Check sheet for the modelled part. Datum: model origin and axes. Units: mm. A direction names the side the tool comes from. Round coordinates to 2 decimals unless told otherwise and drop trailing zeros. Loops run counter-clockwise (first coordinate to the right, second up) from the corner with the lowest first, then second, coordinate; pieces in that order, holes last. Notation, with made-up numbers: (86, -36.5) -> (120, -36.5) arc R25 ccw to (120, -11.5) -> close; hole circle Ø10 at (-0.75, 68.25). An arc over 180 degrees is marked (long way). One line per item, written item: value. Start each with the question number.
1. Go/stop test with flat-tipped pins: pin 1 (4 mm diameter, centred on x = -10.5, y = 9, fed in from -Z); pin 2 (10 mm diameter, centred on x = 7.5, z = -32, fed in from -Y); pin 3 (6 mm diameter, centred on x = -111.5, y = 8.5, fed in from +Z); pin 4 (6.5 mm diameter, centred on x = -91.5, y = 6, fed in from -Z). Record where each tip stops, or that it passes through.
2. Set-up check for faces 1 (the face through (-104, 6, -19.05)), 2 (the face through (104, 6, 19.05)), 3 (the face through (137.218, 6.261, -35.684)): record each of +Z, -Z, +X, -X, +Y, -Y from which the full face is reachable in a straight line by a thin tool's end or side.
3. Cross-section at D-D on x = -16. Record the cut outline in (y, z), then the cut area to 3 significant figures.
4. Cross-section at A-A on z = 23. Record the cut outline in (x, y).
5. Cross-section at B-B on y = 5.25. Record the cut outline in (x, z).
6. Material ranges on L1, parallel to Z at x = -41.5, y = 5.5; L2, parallel to X at y = 11.25, z = 41; L3, parallel to Z at x = 71, y = 8.5, recorded low to high.
7. Release check for a two-part mould opening along X. For faces 4 (the face through (-2, 0, -1)), 5 (the face through (55.31, 6.26, -27.41)), 6 (the face through (152.4, 6, -12)) record: +X half, -X half, draft (parallel to the pull), parting line (faces both ways), or undercut.
8. Cross-section at C-C on z = -23.5. Record the cut outline in (x, y), then the cut area to 3 significant figures.
from build123d import *

# Parameters (mm, degrees)
SKETCH1_R           = 38.1
BOSS_EXTRUDE1_DEPTH = 12.7


with BuildPart() as part:
    # Sketch1 → Boss-Extrude1 (new body)
    with BuildSketch(Plane(origin=(0, 0, 0), x_dir=(1, 0, 0), z_dir=(0, 1, 0))):
        with BuildLine():
            Line((-57.15762, 19.05), (-152.4, 19.05))
            Line((-152.4, 19.05), (-152.4, -44.45))
            Line((-152.4, -44.45), (-121.604136641, -26.67))
            ThreePointArc((-121.604136641, -26.67), (-113.271041312, -18.424847404), (-101.565513762, -17.789517681))
            Line((-101.565513762, -17.789517681), (-7.767081629, -37.301484625))
            ThreePointArc((-7.767081629, -37.301484625), (-37.11967814, -8.620042959), (-23.413788565, 30.062622525))
            ThreePointArc((-23.413788565, 30.062622525), (-39.409915819, 21.872803477), (-57.15762, 19.05))
        make_face()
        with Locations((-0.00762, 0)):
            Circle(SKETCH1_R)
        with BuildLine():
            Line((152.4, -19.05), (152.4, 44.45))
            Line((152.4, 44.45), (121.604136641, 26.67))
            ThreePointArc((121.604136641, 26.67), (113.271041375, 18.424847303), (101.565513804, 17.789517483))
            Line((101.565513804, 17.789517483), (7.750633458, 37.301735929))
            ThreePointArc((7.750633458, 37.301735929), (29.549100528, 24.041844181), (38.09238, 0))
            ThreePointArc((38.09238, 0), (34.18553193, -16.805902567), (23.266219313, -30.165185291))
            ThreePointArc((23.266219313, -30.165185291), (39.319843399, -21.899781819), (57.15, -19.05))
            Line((57.15, -19.05), (152.4, -19.05))
        make_face()
    extrude(amount=BOSS_EXTRUDE1_DEPTH)


solid = part.part
Taken from the geometry:
1. pin 1: stops at z = -37.14
1. pin 2: stops at y = 0
1. pin 3: stops at z = 19.03
1. pin 4: stops at z = -19.05
2. face 1: -Z, -X, +Y, -Y
2. face 2: +Z, +X, +Y, -Y
2. face 3: -Z, +Y, -Y
3. outline: (0, -34.58) -> (12.7, -34.58) -> (12.7, 35.59) -> (0, 35.59) -> close
3. area: 891 mm2
4. outline: (-152.4, 0) -> (-119.31, 0) -> (-119.31, 12.7) -> (-152.4, 12.7) -> close; (-76.52, 0) -> (36.26, 0) -> (36.26, 12.7) -> (-76.52, 12.7) -> close
5. outline: (-152.4, -19.05) -> (-57.16, -19.05) arc R57.2 cw to (-23.41, -30.06) arc R38.1 ccw to (7.75, -37.3) -> (101.57, -17.79) arc R16.51 cw to (121.6, -26.67) -> (152.4, -44.45) -> (152.4, 19.05) -> (57.15, 19.05) arc R57.2 cw to (23.27, 30.17) arc R38.1 ccw to (-7.77, 37.3) -> (-101.57, 17.79) arc R16.51 cw to (-121.6, 26.67) -> (-152.4, 44.45) -> close
6. L1: z = -21.23 to 30.28
6. L2: x = -152.4 to -146.42
6. L3: z = -24.15 to 19.05
7. face 4: draft
7. face 5: undercut
7. face 6: +X half
8. outline: (-35.04, 0) -> (74.11, 0) -> (74.11, 12.7) -> (-35.04, 12.7) -> close; (119.7, 0) -> (152.4, 0) -> (152.4, 12.7) -> (119.7, 12.7) -> close
8. area: 1,800 mm2
